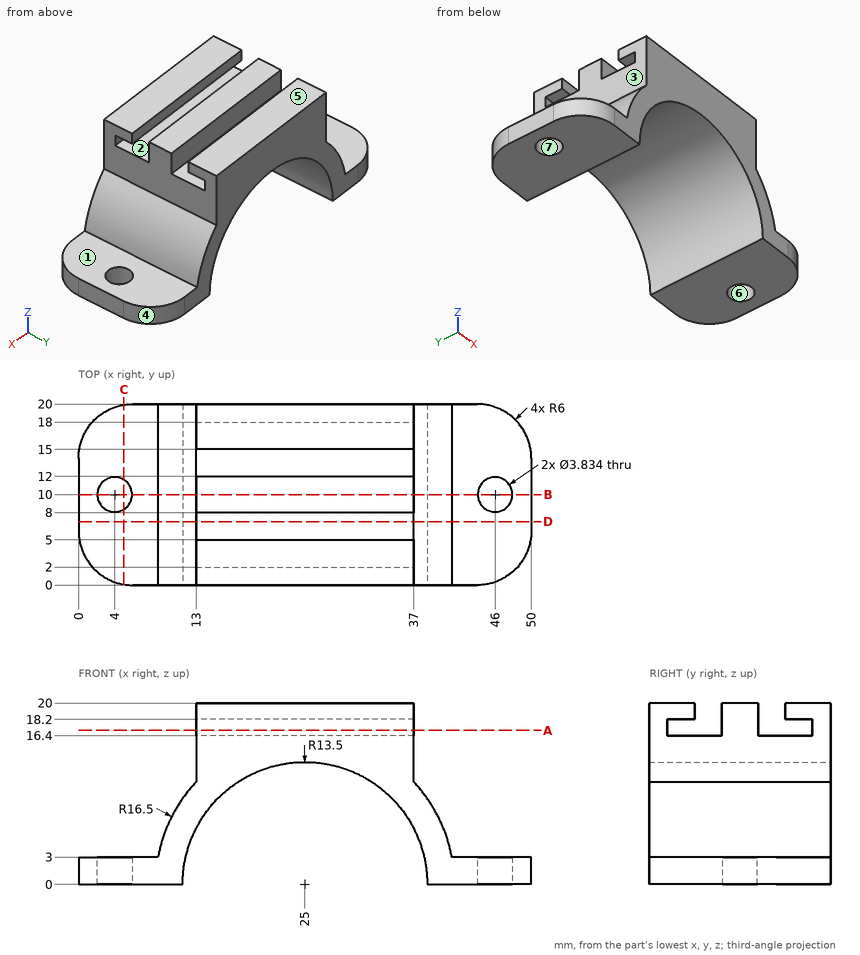
Check sheet for the drawn part. Datum: minimum x, y, z corner. Units: mm. A direction names the side the tool comes from. Give positions to 0.01 mm unless a question says otherwise; leave off trailing zeros. Order: outer loops, then holes, each group sorted by start corner. A loop starts at its lowest first (then second) coordinate and runs counter-clockwise, first axis right, second up. Notation, with made-up numbers: (41.25, 52.25) - (74.25, 52.25) arc R8 cw to (74.25, 67.25) - close; hole circle Ø11 at (60.25, 89). An arc over 180 degrees is marked (long way). Answer in a Markdown table with one row per item. Add a question column.
Q1. Cross-section at A-A, the plane z = 17. Enter the section's corners in (x, y), then the cut area to 3 significant figures.
Q2. Mould release check, pull along X, two halves, no side actions. Record for the marked faces 4, 5, 6 and 7: pulls with the +X half, pulls with the -X half, needs draft (parallel to the pull), parting line crosses it, or undercut.
Q3. Tool access check on the marked faces 1, 2 and 3. Record the directions out of +Z, -Z, +X, -X, +Y, -Y that give a thin tool (end or side, any length) a straight path to the whole face; none if there is none.
Q4. Cross-section at D-D, the plane y = 7. Enter the section's corners in (x, z) (1 decimal), then the cut area to 3 significant figures.
Q5. Cross-section at B-B, the plane y = 10. Enter the section's corners in (x, z) (1 decimal), then the cut area to 3 significant figures.
Q6. Gauge pin test, flat ends, axial feed: pin 1 (4.5 mm diameter, centred on x = 46, y = 10, fed in from +Z); pin 2 (5 mm diameter, centred on y = 7, z = 13.5, fed in from -X); pin 3 (2.5 mm diameter, centred on x = 4, y = 10, fed in from +Z); pin 4 (1.5 mm diameter, centred on y = 4.5, z = 2.5, fed in from +X). Record the tip position at first contact, or that the pin passes through.
Q7. Material ranges on probe 1 along Y at (x, z) = (26.5, 17.25); probe 2 along Z at (x, y) = (24.5, 3); probe 3 along Z at (x, y) = (42.5, 15), recorded low to high. Write a range as from..to.
Q8. Cross-section at C-C, the plane x = 5. Enter the section's corners in (y, z).
Check values:
| question | item | result |
|---|---|---|
| 1 | outline | (13, 0) - (37, 0) - (37, 2) - (13, 2) - close; (13, 8) - (37, 8) - (37, 12) - (13, 12) - close; (13, 18) - (37, 18) - (37, 20) - (13, 20) - close |
| 1 | area | 192 mm^2 |
| 2 | face 4 | pulls with the +X half |
| 2 | face 5 | needs draft |
| 2 | face 6 | undercut |
| 2 | face 7 | undercut |
| 3 | face 1 | +Z, +X, +Y, -Y |
| 3 | face 2 | +X, -X |
| 3 | face 3 | +Z, -X, +Y, -Y |
| 4 | outline | (0, 0) - (11.5, 0) arc R13.5 cw to (38.5, 0) - (50, 0) - (50, 3) - (41.2, 3) arc R16.5 ccw to (37, 11.3) - (37, 16.4) - (13, 16.4) - (13, 11.3) arc R16.5 ccw to (8.8, 3) - (0, 3) - close |
| 4 | area | 229 mm^2 |
| 5 | outline | (0, 0) - (2.1, 0) - (2.1, 3) - (0, 3) - close; (5.9, 0) - (11.5, 0) arc R13.5 cw to (38.5, 0) - (44.1, 0) - (44.1, 3) - (41.2, 3) arc R16.5 ccw to (37, 11.3) - (37, 20) - (13, 20) - (13, 11.3) arc R16.5 ccw to (8.8, 3) - (5.9, 3) - close; (47.9, 0) - (50, 0) - (50, 3) - (47.9, 3) - close |
| 5 | area | 292 mm^2 |
| 6 | pin 1 | stops at z = 3 |
| 6 | pin 2 | stops at x = 12.7 |
| 6 | pin 3 | passes through |
| 6 | pin 4 | stops at x = 49.95 |
| 7 | probe 1 | y = 0..2, 8..12, 18..20 |
| 7 | probe 2 | z = 13.49..16.4, 18.2..20 |
| 7 | probe 3 | z = 0..3 |
| 8 | outline | (0.08, 0) - (8.36, 0) - (8.36, 3) - (0.08, 3) - close; (11.64, 0) - (19.92, 0) - (19.92, 3) - (11.64, 3) - close |
